The listing builds one solid part. Answer for the finished solid, in the listing's coordinates (mm). A direction names the side the tool comes from. Give positions to 0.01 mm unless a question says otherwise; leave off trailing zeros. Order: outer loops, then holes, each group sorted by start corner. A loop starts at its lowest first (then second) coordinate and runs counter-clockwise, first axis right, second up. Notation, with made-up numbers: (61.25, -26) - (116.25, -26) arc R12 ccw to (116.25, -13) - close; hole circle Ø3 at (-34, 55). An arc over 180 degrees is marked (long way). Answer as a JSON object with one key per item and string values. Group by question number.
Q1. For faces 4 (the face through (11, 29.1, -21)), 5 (the face through (-25.05, 14.35, 0.19)), determine the directions among +Z, -Z, +X, -X, +Y, -Y from which every point of the face is accessible in a straight line to the end or side of a thin tool.
Q2. Given pin 1 (3 mm diameter, centred on x = -26.5, z = 36.5, fed in from -Y); pin 2 (6 mm diameter, centred on x = -2, y = 11.5, fed in from -Z); pin 3 (1 mm diameter, centred on x = 36.5, y = 9.5, fed in from +Z); pin 4 (6 mm diameter, centred on y = 5, z = 8, fed in from +X), each flat-ended and moving along its own axis, determine where each tip first touches the part or whether it passes through.
Q3. A cutting plane is placed at D-D, the plane z = -33. Give the vertices of the cut face in (x, y).
Q4. A cutting plane is placed at A-A, the plane x = -22. Give the vertices of the cut face in (y, z), and give its area (3 significant figures).
Q5. Consider line 1 (X direction, y = 5, z = 15); line 2 (Z direction, x = 11.5, y = 16); line 3 (Z direction, x = 9, y = 26.5). Determine where each line is inside the solid, lowest interval first.
Q6. The mould has two halves that part along Z. Classify faces 1 (the face through (22.5, 14.3, -0.2)), 2 (the face through (11, 0, -21)), 3 (the face through (47.954, 14.346, -2.11)): released by +Z, released by -Z, zero draft, split by the parting line, or undercut.
Q7. A cutting plane is placed at C-C, the plane y = 6.5. Give the vertices of the cut face in (x, z).
Q8. A cutting plane is placed at B-B, the plane z = 0. Give the vertices of the cut face in (x, y), and give its area (3 significant figures).
Autodesk Inventor part; units mm, degrees
ref_plane "YZ Plane" through (0, 0, 0) normal (1, 0, 0) x (0, 1, 0)
ref_plane "XZ Plane" through (0, 0, 0) normal (0, 1, 0) x (-1, 0, 0)
ref_plane "XY Plane" through (0, 0, 0) normal (0, 0, 1) x (1, 0, 0)
sketch "Sketch1" plane through (0, 0, 0) normal (0, 1, 0) x (-1, 0, 0)
  circle A0 centre (0, 0) radius 48
  dimension "d0" = 96
extrude "Extrusion1" add sketch "Sketch1" along normal blind 29.1
sketch "Sketch2" plane through (0, 29.1, 0) normal (0, 1, 0) x (1, 0, 0)
  point P0 (0, 0)
  point P1 (-2.5528, 0.0324)
hole "Hole1" at (-2.5528, 29.1, -0.0324) direction (0, -1, 0) diameter 45 end through all
sketch "Sketch3" plane through (0, 29.1, 0) normal (0, 1, 0) x (1, 0, 0)
  point P0 (0, 0)
sketch "Sketch4" plane through (0, 29.1, 0) normal (0, 1, 0) x (1, 0, 0)
  point P0 (0, 0)
hole "Hole2" at (0, 29.1, 0) direction (0, -1, 0) diameter 45 end through all
properties part number "bobina_sin_numero"
Reply:
{
 "1": {"face 4": "+Z, -Z, +X, -X, +Y", "face 5": "+Y, -Y"},
 "2": {"pin 1": "stops at y = 0", "pin 2": "stops at z = -48", "pin 3": "stops at z = 31.75", "pin 4": "stops at x = 47.74"},
 "3": {"outline": "(-34.86, 0) - (34.86, 0) - (34.86, 29.1) - (-34.86, 29.1) - close"},
 "4": {"outline": "(0, -42.66) - (29.1, -42.66) - (29.1, -11.35) - (0, -11.35) - close; (0, 11.28) - (29.1, 11.28) - (29.1, 42.66) - (0, 42.66) - close", "area": "1,820 mm^2"},
 "5": {"line 1": "x = -45.6 to -19.29, 16.77 to 45.6", "line 2": "z = -46.6 to -19.34, 19.34 to 46.6", "line 3": "z = -47.15 to -20.62, 20.62 to 47.15"},
 "6": {"face 1": "undercut", "face 2": "zero draft", "face 3": "split by the parting line"},
 "7": {"outline": "circle Ø96 at (0, 0); hole (-1.56, 22.45) arc R22.5 ccw (long way) to (-0.99, -22.48) arc R22.5 ccw (long way) to start"},
 "8": {"outline": "(-48, 0) - (-25.05, 0) - (-25.05, 29.1) - (-48, 29.1) - close; (22.5, 0) - (48, 0) - (48, 29.1) - (22.5, 29.1) - close", "area": "1,410 mm^2"}
}
